Part model, mm, in its own coordinate system. A direction names the side the tool comes from. Round coordinates to 2 decimals unless told otherwise and drop trailing zeros. Use a Markdown table: item, result. Add a question column.
1) Wall check: probe 1 along Y at (x, z) = (0, 30.5) (3 decimals); probe 2 along X at (y, z) = (6, 4.5); probe 3 along Y at (x, z) = (0, 29) (3 decimals). Give the ranges that are in metal, low to high.
2) Drop flat-ended pins along their axis: P1, Ø1, axis at y = 50, z = 23, coming from the -X side; P2, Ø10, axis at x = 8.5, z = 15, coming from the -Y side; P3, Ø2, axis at x = 27, z = 14, coming from the -Y side. Give the stop position or say it passes through.
3) Slice it at A-A on x = 0. Give the number of separate pieces and of enclosed holes in the cut face, plus the area to 3 significant figures.
4) Two-plate mould, pull along Y, no slides. Class faces 5 (the face through (45.2, 44.37, 10.15)), 6 (the face through (-45, 25, 41)), 7 (the face through (-2.64, -66.623, 20.213)): released by +Y, released by -Y, zero draft, split by the parting line, or undercut.
5) Which spindle directions (+Z, -Z, +X, -X, +Y, -Y) get a long thin tool onto all of the face, cutting with end or side? Do faces 1 (the face through (-23, 1, 4)), 2 (the face through (14, 1, 0)), 3 (the face through (-40, 40, 6.075)), 4 (the face through (9, 64.375, 24)). Say none if no direction does.
```python
from build123d import *

# Parameters (mm, degrees)
SKETCH031_R           = 66.675
PAD006_DEPTH          = 41
SKETCH032_W           = 41
SKETCH032_H           = 10
PAD007_DEPTH          = 41
SKETCH033_R           = 8.75
POCKET048_DEPTH       = 16
SKETCH034_W           = 25.5
SKETCH034_H           = 25.5
POCKET049_DEPTH       = 2.3
SKETCH035_R           = 1.7
POCKET050_DEPTH       = 16
POCKET051_DEPTH       = 37
SKETCH037_R           = 1.6
POCKET052_DEPTH       = 446.937769
POLARPATTERN017_COUNT = 4
POCKET053_DEPTH       = 30
POLARPATTERN018_COUNT = 4
SKETCH040_R           = 50.675
POCKET054_DEPTH       = 37
SKETCH041_R           = 3.675
POCKET055_DEPTH       = 426.98258
POLARPATTERN019_COUNT = 3
SKETCH042_R           = 22.5
PAD013_DEPTH          = 2
SKETCH044_R           = 7.25
POCKET056_DEPTH       = 6.001
SKETCH045_W           = 28
SKETCH045_H           = 10
POCKET057_DEPTH       = 37
CHAMFER008_SIZE       = 1


with BuildPart() as part:
    # Sketch031 → Pad006 (new body)
    with BuildSketch(Plane.XY):
        Circle(SKETCH031_R)
    extrude(amount=PAD006_DEPTH)

    # Sketch032 (on Face3 of Pad006) → Pad007 (join)
    with BuildSketch(Plane.XY.offset(41)):
        with Locations((0, 61.675)):
            Rectangle(SKETCH032_W, SKETCH032_H)
    extrude(amount=-PAD007_DEPTH)

    # Sketch033 (on Face8 of Pad007) → Pocket048 (cut)
    with BuildSketch(Plane(origin=(0, 66.675, 0), x_dir=(-1, 0, 0), z_dir=(0, 1, 0))):
        with Locations((0, 20.5)):
            Circle(SKETCH033_R)
    extrude(amount=-POCKET048_DEPTH, mode=Mode.SUBTRACT)

    # Sketch034 (on Face8 of Pocket048) → Pocket049 (cut)
    with BuildSketch(Plane(origin=(0, 66.675, 0), x_dir=(-1, 0, 0), z_dir=(0, 1, 0))):
        with Locations((0, 20.5)):
            Rectangle(SKETCH034_W, SKETCH034_H)
    extrude(amount=-POCKET049_DEPTH, mode=Mode.SUBTRACT)

    # Sketch035 (on Face19 of Pocket049) → Pocket050 (cut)
    with BuildSketch(Plane(origin=(0, 64.375, 0), x_dir=(-1, 0, 0), z_dir=(0, 1, 0))):
        with Locations((-9.1, 29.6)):
            Circle(SKETCH035_R)
        with Locations((9.1, 29.6)):
            Circle(SKETCH035_R)
        with Locations((9.1, 11.4)):
            Circle(SKETCH035_R)
        with Locations((-9.1, 11.4)):
            Circle(SKETCH035_R)
    extrude(amount=-POCKET050_DEPTH, mode=Mode.SUBTRACT)

    # Sketch036 → Pocket051 (cut)
    with BuildSketch(Plane.XY.offset(41)):
        Polygon((0, 47.1465), (-47.146189, 0), (0, -47.1465), (47.146189, 0), align=None)
    extrude(amount=-POCKET051_DEPTH, mode=Mode.SUBTRACT)

    # Sketch037 (on Face13 of Pocket051) → Pocket052 (cut, through all)
    with BuildSketch(Plane(origin=(23.57325, -23.573095, 0), x_dir=(-0.707104, -0.707109, 0), z_dir=(-0.707109, 0.707104, 0))):
        with Locations((0, 8.5)):
            Circle(SKETCH037_R)
    pocket052 = extrude(amount=-POCKET052_DEPTH, mode=Mode.SUBTRACT)

    # PolarPattern017: Pocket052 ×4 about axis
    polarpattern017_axis = Axis((0, 0, 0), (0, 0, 1))
    for i in range(1, POLARPATTERN017_COUNT):
        add(pocket052.rotate(polarpattern017_axis, i * 360 / POLARPATTERN017_COUNT), mode=Mode.SUBTRACT)

    # Sketch039 (on Face18 of PolarPattern017) → Pocket053 (cut)
    with BuildSketch(Plane(origin=(23.57325, -23.573095, 0), x_dir=(-0.707104, -0.707109, 0), z_dir=(-0.707109, 0.707104, 0))):
        Polygon((2.8, 8.5), (1.4, 10.924871), (-1.4, 10.924871), (-2.8, 8.5), (-1.4, 6.075129), (1.4, 6.075129), align=None)
    pocket053 = extrude(amount=-POCKET053_DEPTH, mode=Mode.SUBTRACT)

    # PolarPattern018: Pocket053 ×4 about axis
    polarpattern018_axis = Axis((0, 0, 0), (0, 0, 1))
    for i in range(1, POLARPATTERN018_COUNT):
        add(pocket053.rotate(polarpattern018_axis, i * 360 / POLARPATTERN018_COUNT), mode=Mode.SUBTRACT)

    # Sketch040 → Pocket054 (cut)
    with BuildSketch(Plane.XY.offset(41)):
        Circle(SKETCH040_R)
    extrude(amount=-POCKET054_DEPTH, mode=Mode.SUBTRACT)

    # Sketch041 → Pocket055 (cut, through all)
    with BuildSketch(Plane.XY.offset(41)):
        with Locations((0, -58.675)):
            Circle(SKETCH041_R)
    pocket055 = extrude(amount=-POCKET055_DEPTH, mode=Mode.SUBTRACT)

    # PolarPattern019: Pocket055 ×3 about axis
    polarpattern019_axis = Axis((0, 0, 41), (0, 0, 1))
    for i in range(1, POLARPATTERN019_COUNT):
        add(pocket055.rotate(polarpattern019_axis, i * 360 / POLARPATTERN019_COUNT), mode=Mode.SUBTRACT)

    # Sketch042 (on Face61 of PolarPattern019) → Pad013 (join)
    with BuildSketch(Plane.XY.offset(4)):
        Circle(SKETCH042_R)
    extrude(amount=PAD013_DEPTH)

    # Sketch044 (on Face66 of Pad013) → Pocket056 (cut, through all)
    with BuildSketch(Plane.XY.offset(6)):
        Circle(SKETCH044_R)
    extrude(amount=-POCKET056_DEPTH, mode=Mode.SUBTRACT)

    # Sketch045 (on Face5 of Pocket056) → Pocket057 (cut)
    with BuildSketch(Plane.XY.offset(41)):
        with Locations((0, 47)):
            Rectangle(SKETCH045_W, SKETCH045_H)
    extrude(amount=-POCKET057_DEPTH, mode=Mode.SUBTRACT)

    # Chamfer008
    chamfer008_edges = [part.edges().sort_by_distance(p)[0] for p in [
        (-22.5, 0, 6),
    ]]
    chamfer(chamfer008_edges, length=CHAMFER008_SIZE)


solid = part.part
```
Entries:
| question | item | result |
|---|---|---|
| 1 | probe 1 | y = -66.675 to -62.35, -55 to -50.675, 52 to 64.375 |
| 1 | probe 2 | x = -66.4 to -50.32, -21.69 to -4.07, 4.07 to 21.69, 50.32 to 66.4 |
| 1 | probe 3 | y = -66.675 to -62.35, -55 to -50.675 |
| 2 | P1 | stops at x = -44.67 |
| 2 | P2 | stops at y = -66.58 |
| 2 | P3 | stops at y = -61.4 |
| 3 | separate pieces | 4 |
| 3 | enclosed holes | 0 |
| 3 | area | 1,090 mm^2 |
| 4 | face 5 | undercut |
| 4 | face 6 | zero draft |
| 4 | face 7 | split by the parting line |
| 5 | face 1 | +Z |
| 5 | face 2 | -Z, +X, -X, +Y, -Y |
| 5 | face 3 | none |
| 5 | face 4 | +Y |
